from build123d import *

# Parameters (mm, degrees)
SKETCH_2_R      = 1.5
SKETCH_2_R_2    = 1
EXTRUDE_1_DEPTH = 2
FILLET_1_R      = 7


with BuildPart() as part:
    # 草圖2 → 填料-伸長1 (new body)
    with BuildSketch(Plane(origin=(0, 0, 0), x_dir=(-1, 0, 0), z_dir=(0, 1, 0))):
        Polygon((23.696699141, -31.196699141), (-23.696699141, -31.196699141), (-35.696699141, -31.196699141), (-35.696699141, -19.196699141), (-35.696699141, 19.196699141), (-35.696699141, 31.196699141), (-23.696699141, 31.196699141), (23.696699141, 31.196699141), (35.696699141, 31.196699141), (35.696699141, 19.196699141), (35.696699141, -19.196699141), (35.696699141, -31.196699141), align=None)
        with Locations((29, 24.5)):
            Circle(SKETCH_2_R, mode=Mode.SUBTRACT)
        with Locations((29, -24.5)):
            Circle(SKETCH_2_R, mode=Mode.SUBTRACT)
        with Locations((-29, 24.5)):
            Circle(SKETCH_2_R, mode=Mode.SUBTRACT)
        with Locations((-29, -24.5)):
            Circle(SKETCH_2_R, mode=Mode.SUBTRACT)
        with Locations((5.699998849, -24.700000266)):
            Circle(SKETCH_2_R_2, mode=Mode.SUBTRACT)
        with Locations((-5.700001151, 24.699999734)):
            Circle(SKETCH_2_R_2, mode=Mode.SUBTRACT)
        with BuildLine():
            Line((23.696699141, -22.196699141), (10.359084004, -22.196699141))
            ThreePointArc((10.359084004, -22.196699141), (9.135687554, -22.005019128), (8.029541427, -21.448349703))
            ThreePointArc((8.029541427, -21.448349703), (5.699998849, -20.700000266), (3.370456271, -21.448349703))
            ThreePointArc((3.370456271, -21.448349703), (2.264310144, -22.005019128), (1.040913694, -22.196699141))
            Line((1.040913694, -22.196699141), (-23.696699141, -22.196699141))
            ThreePointArc((-23.696699141, -22.196699141), (-25.818019485, -21.318019485), (-26.696699141, -19.196699141))
            Line((-26.696699141, -19.196699141), (-26.696699141, 19.196699141))
            ThreePointArc((-26.696699141, 19.196699141), (-25.818019485, 21.318019485), (-23.696699141, 22.196699141))
            Line((-23.696699141, 22.196699141), (-10.359087048, 22.196699141))
            ThreePointArc((-10.359087048, 22.196699141), (-9.13569038, 22.005019059), (-8.029544099, 21.448349438))
            ThreePointArc((-8.029544099, 21.448349438), (-5.700001151, 20.699999734), (-3.370458203, 21.448349438))
            ThreePointArc((-3.370458203, 21.448349438), (-2.264311922, 22.005019059), (-1.040915254, 22.196699141))
            Line((-1.040915254, 22.196699141), (23.696699141, 22.196699141))
            ThreePointArc((23.696699141, 22.196699141), (25.818019485, 21.318019485), (26.696699141, 19.196699141))
            Line((26.696699141, 19.196699141), (26.696699141, -19.196699141))
            ThreePointArc((26.696699141, -19.196699141), (25.818019485, -21.318019485), (23.696699141, -22.196699141))
        make_face(mode=Mode.SUBTRACT)
    extrude(amount=EXTRUDE_1_DEPTH)

    # 圓角1
    fillet_1_edges = [part.edges().sort_by_distance(p)[0] for p in [
        (35.696699141, 1, -31.196699141),
        (35.696699141, 1, 31.196699141),
        (-35.696699141, 1, 31.196699141),
        (-35.696699141, 1, -31.196699141),
    ]]
    fillet(fillet_1_edges, radius=FILLET_1_R)


solid = part.part
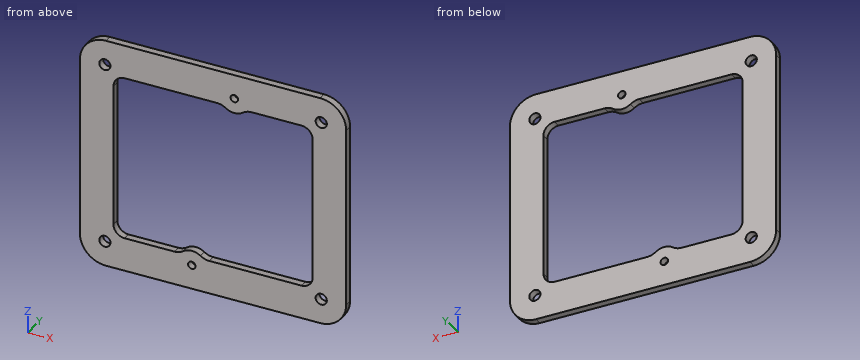
Here's how the part is built. I have some questions about the finished solid (model axes, mm). Give positions to 0.01 mm unless a question says otherwise; leave off trailing zeros. Order: outer loops, then holes, each group sorted by start corner. A loop starts at its lowest first (then second) coordinate and runs counter-clockwise, first axis right, second up. Notation, with made-up numbers: M -23,41 L -13,41 A26 ccw -13,76 Z; hole C 26,73.5 d2. An arc over 180 degrees is marked long. Answer as a JSON object with one key per item and string values. Group by question number.
1) Suppose I cut it at A-A, the plane x = -20. Write out the boundary of the cut face in (y, z).
2) Please list where these lines run through material, in increasing order: L1, parallel to Z at x = -29, y = 1.15; L2, parallel to X at y = 1.6, z = -0.5; L3, parallel to Z at x = -10.5, y = 1.3. Write a range as [from, to].
3) Suppose I cut it at B-B, the plane y = 1.4. Count the separate pieces of the cut face and the enclosed holes in it, plus the area to 3 significant figures.
4) Suppose I cut it at C-C, the plane z = 8. Write out the boundary of the cut face in (x, y), plus the area to 3 significant figures.
Results found:
{
 "1": {"outline": "M 0,-31.2 L 2,-31.2 L 2,-22.2 L 0,-22.2 Z; M 0,22.2 L 2,22.2 L 2,31.2 L 0,31.2 Z"},
 "2": {"L1": "[-31.19, -26], [-23, 23], [26, 31.19]", "L2": "[-35.7, -26.7], [26.7, 35.7]", "L3": "[-31.2, -22.2], [22.2, 31.2]"},
 "3": {"separate pieces": "1", "enclosed holes": "7", "area": "2,030 mm²"},
 "4": {"outline": "M -35.7,0 L -26.7,0 L -26.7,2 L -35.7,2 Z; M 26.7,0 L 35.7,0 L 35.7,2 L 26.7,2 Z", "area": "36.0 mm²"}
}
